Design review of the part shown in the three views and the two pictorial views. Dimensions are in mm from the part's minimum x, y and z. Give positions to 0.01 mm unless a question says otherwise; leave off trailing zeros. Loops run counter-clockwise (first coordinate to the right, second up) from the corner with the lowest first, then second, coordinate; pieces in that order, holes last. Notation, with made-up numbers: M 85,-38.75 L 126,-38.75 A24 ccw 126,0.25 Z; hole C 81.25,-2.5 d5. An arc over 180 degrees is marked long. Return JSON: item names as keys, results as strings. Group by question number.
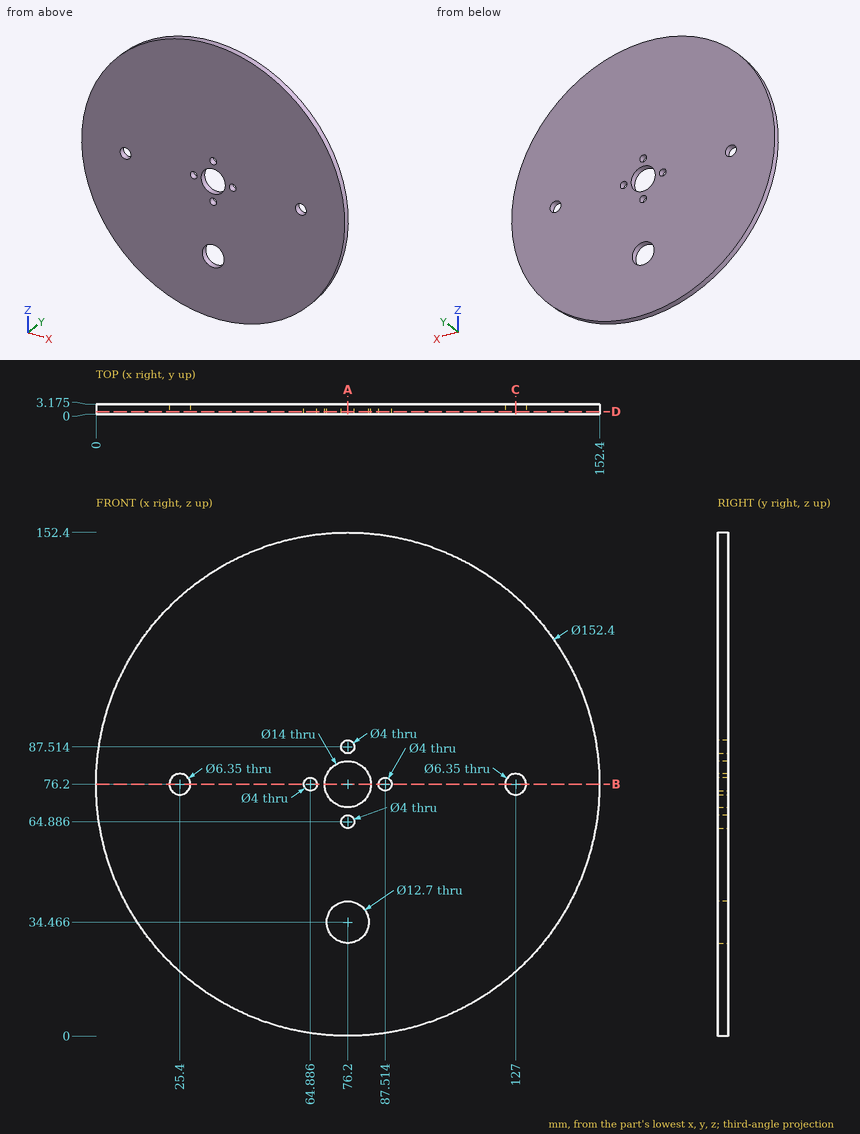
(1) Add section C-C (x = 127). Write out the cut boundary in (y, z) (3 decimals).
(2) Add section A-A (x = 76.2). Write out the cut boundary in (y, z) (1 decimal).
(3) Add section D-D (y = 0.9). Count the separate pieces of the cut face and the enclosed holes in it, and give its area (3 significant figures).
(4) For pin 1 (2.5 mm diameter, centred on x = 87.514, z = 76.2, fed in from -Y); pin 2 (5 mm diameter, centred on x = 76.2, z = 64.886, fed in from +Y) (3 decimals), all flat-tipped, find the tip position at first contact; note any pin that passes through.
(5) Add section B-B (z = 76.2). Write out the cut boundary in (x, y) (3 decimals), and give its area (3 significant figures).
(6) For probe 1 along X at (y, z) = (1.4, 76.2) (3 decimals); probe 2 along Z at (x, y) = (71, 1.5) (1 decimal); probe 3 along Z at (x, y) = (71.5, 2.8) (1 decimal), list the stretches that pass through material, from the lowest coordinate up.
Verdict:
{
 "1": {"outline": "M 0,19.404 L 3.175,19.404 L 3.175,73.025 L 0,73.025 Z; M 0,79.375 L 3.175,79.375 L 3.175,132.996 L 0,132.996 Z"},
 "2": {"outline": "M 0,0 L 3.2,0 L 3.2,28.1 L 0,28.1 Z; M 0,40.8 L 3.2,40.8 L 3.2,62.9 L 0,62.9 Z; M 0,66.9 L 3.2,66.9 L 3.2,69.2 L 0,69.2 Z; M 0,83.2 L 3.2,83.2 L 3.2,85.5 L 0,85.5 Z; M 0,89.5 L 3.2,89.5 L 3.2,152.4 L 0,152.4 Z"},
 "3": {"separate pieces": "1", "enclosed holes": "8", "area": "17,800 mm²"},
 "4": {"pin 1": "passes through", "pin 2": "stops at y = 3.175"},
 "5": {"outline": "M 0,0 L 22.225,0 L 22.225,3.175 L 0,3.175 Z; M 28.575,0 L 62.886,0 L 62.886,3.175 L 28.575,3.175 Z; M 66.886,0 L 69.2,0 L 69.2,3.175 L 66.886,3.175 Z; M 83.2,0 L 85.514,0 L 85.514,3.175 L 83.2,3.175 Z; M 89.514,0 L 123.825,0 L 123.825,3.175 L 89.514,3.175 Z; M 130.175,0 L 152.4,0 L 152.4,3.175 L 130.175,3.175 Z", "area": "374 mm²"},
 "6": {"probe 1": "x = 0 to 22.225, 28.575 to 62.886, 66.886 to 69.2, 83.2 to 85.514, 89.514 to 123.825, 130.175 to 152.4", "probe 2": "z = 0.2 to 30.8, 38.1 to 71.5, 80.9 to 152.2", "probe 3": "z = 0.1 to 30.2, 38.7 to 71, 81.4 to 152.3"}
}
